from build123d import *

# Parameters (mm, degrees)
EXTRUDE_1_DEPTH     = 2
SKETCH_2_R          = 2
SKETCH_2_R_2        = 1.9
CUT_EXTRUDE_1_DEPTH = 3
CUT_EXTRUDE_2_DEPTH = 3
SKETCH_4_R          = 1.75
CUT_EXTRUDE_3_DEPTH = 3


with BuildPart() as part:
    # 草图1 → 凸台-拉伸1 (new body)
    with BuildSketch(Plane.XY):
        with BuildLine():
            Line((-47, 40), (47, 40))
            ThreePointArc((47, 40), (49.121320344, 39.121320344), (50, 37))
            Line((50, 37), (50, -37))
            ThreePointArc((50, -37), (49.121320344, -39.121320344), (47, -40))
            Line((47, -40), (-47, -40))
            ThreePointArc((-47, -40), (-49.121320344, -39.121320344), (-50, -37))
            Line((-50, -37), (-50, 37))
            ThreePointArc((-50, 37), (-49.121320344, 39.121320344), (-47, 40))
        make_face()
    extrude(amount=EXTRUDE_1_DEPTH)

    # 草图2 → 切除-拉伸1 (cut, through all)
    with BuildSketch(Plane.XY.offset(2)):
        with Locations((-46.8, 36.8)):
            Circle(SKETCH_2_R)
        with Locations((46.8, 36.8)):
            Circle(SKETCH_2_R)
        with Locations((46.8, -36.8)):
            Circle(SKETCH_2_R)
        with Locations((-46.8, -36.8)):
            Circle(SKETCH_2_R)
        with Locations((-43, 29)):
            Circle(SKETCH_2_R)
        with Locations((6, 29)):
            Circle(SKETCH_2_R)
        with Locations((6, -29)):
            Circle(SKETCH_2_R)
        with Locations((-43, -29)):
            Circle(SKETCH_2_R)
        with Locations((47, -15)):
            Circle(SKETCH_2_R_2)
        with Locations((20, 15)):
            Circle(SKETCH_2_R_2)
        with Locations((20, -15)):
            Circle(SKETCH_2_R_2)
        with Locations((47, 15)):
            Circle(SKETCH_2_R_2)
    extrude(amount=-CUT_EXTRUDE_1_DEPTH, mode=Mode.SUBTRACT)

    # 草图3 → 切除-拉伸2 (cut, through all)
    with BuildSketch(Plane.XY.offset(2)):
        with BuildLine():
            Line((26, 33.8), (38, 33.8))
            ThreePointArc((38, 33.8), (41.8, 30), (38, 26.2))
            Line((38, 26.2), (26, 26.2))
            ThreePointArc((26, 26.2), (22.2, 30), (26, 33.8))
        make_face()
    extrude(amount=-CUT_EXTRUDE_2_DEPTH, mode=Mode.SUBTRACT)

    # 草图4 → 切除-拉伸3 (cut, through all)
    with BuildSketch(Plane.XY.offset(2)):
        with Locations((-37.5, 0.169558906)):
            Circle(SKETCH_4_R)
        with Locations((37.5, 0)):
            Circle(SKETCH_4_R)
    extrude(amount=-CUT_EXTRUDE_3_DEPTH, mode=Mode.SUBTRACT)


solid = part.part
Check sheet for the modelled part. Datum: model origin and axes. Units: mm. A direction names the side the tool comes from. Give positions to 0.01 mm unless a question says otherwise; leave off trailing zeros. Answer as CSV lines item,"result". Start each with the question number.
Item 1: Thickness scan on line 1 (Y direction, x = 47, z = 1.1); line 2 (Y direction, x = 20, z = 0.75); line 3 (Y direction, x = -43, z = 1.25). Record the ranges inside material, lowest first. Write a range as [from, to].
Item 2: Tool access check on faces 1 (the face through (50, 1, 1)), 2 (the face through (32, 33.8, 1)). Record the directions out of +Z, -Z, +X, -X, +Y, -Y that give a thin tool (end or side, any length) a straight path to the whole face; none if there is none.
Item 3: Cross-section at A-A on z = 0.75. State how many separate pieces and enclosed holes the cut face has, plus the area to 3 significant figures.
Item 4: Mould release check, pull along Y, two halves, no side actions. Record for faces 3 (the face through (1, 1, 2)), 4 (the face through (1, -40, 1)), 5 (the face through (32, 26.2, 1)): +Y half, -Y half, draft (parallel to the pull), parting line (faces both ways), or undercut.
Item 5: Gauge pin test, flat end, axial feed: P1, Ø3, axis at x = -43, y = -29, coming from the -Z side. Record the tip position at first contact, or that the pin passes through.
Established:
1,line 1,"y = [-40, -38.79], [-34.81, -16.9], [-13.1, 13.1], [16.9, 34.81], [38.79, 40]"
1,line 2,"y = [-40, -16.9], [-13.1, 13.1], [16.9, 40]"
1,line 3,"y = [-40, -31], [-27, 27], [31, 40]"
2,face 1,"+Z, -Z, +X, +Y, -Y"
2,face 2,"+Z, -Z"
3,separate pieces,"1"
3,enclosed holes,"15"
3,area,"7,690 mm^2"
4,face 3,"draft"
4,face 4,"-Y half"
4,face 5,"undercut"
5,P1,"passes through"
